The listing builds one solid part. Answer for the finished solid, in the listing's coordinates (mm). A direction names the side the tool comes from. Give positions to 0.01 mm unless a question says otherwise; leave off trailing zeros. Loops run counter-clockwise (first coordinate to the right, second up) from the corner with the lowest first, then second, coordinate; pieces in that order, holes last. Notation, with made-up numbers: (54.25, 56) - (63.25, 56) arc R17 ccw to (63.25, 87) - close; hole circle Ø4 at (25, 73). An arc over 180 degrees is marked (long way). One line per item, written item: value. Start each with the question number.
from build123d import *

# Parameters (mm, degrees)
FILLET1_R    = 1.3
SKETCH3_W    = 1.03
SKETCH3_H    = 4.9
SKETCH4_W    = 1.03
SKETCH4_H    = 1.858652296
RECPAT_COUNT = 2
RECPAT_ANGLE = 90


with BuildPart() as part:
    # BodySke → Base-Revolve (revolve)
    with BuildSketch(Plane.XY):
        Polygon((0, 0), (0, 4.65), (0.55, 4.65), (2.7, 2.5), (40, 2.5), (40, 0), align=None)
    revolve(axis=Axis((-6.35, 0, 0), (1, 0, 0)))

    # Fillet1
    fillet1_edges = [part.edges().sort_by_distance(p)[0] for p in [
        (2.7, -2.5, 0),
    ]]
    fillet(fillet1_edges, radius=FILLET1_R)

    # Sketch3 → Recess section 0
    with BuildSketch(Plane.ZY):
        Rectangle(SKETCH3_W, SKETCH3_H)
    # Sketch4 → Recess section 1
    with BuildSketch(Plane.ZY.offset(-3.05)):
        Rectangle(SKETCH4_W, SKETCH4_H)
    recess = loft(mode=Mode.SUBTRACT)

    # RecPat: Recess ×2 about axis
    recpat_axis = Axis((0, 0, 0), (1, 0, 0))
    for i in range(1, RECPAT_COUNT):
        add(recess.rotate(recpat_axis, i * RECPAT_ANGLE / (RECPAT_COUNT - 1)), mode=Mode.SUBTRACT)

    # RecCorSke → RecessCore (revolve, cut)
    with BuildSketch(Plane.XY):
        Polygon((0, 0), (0, 1.064276776), (3.05, 0.851), (3.326506661, 0), align=None)
    revolve(axis=Axis((-3.175, 0, 0), (1, 0, 0)), mode=Mode.SUBTRACT)


solid = part.part
1. A cutting plane is placed at A-A (x = 33). Determine the outline of the cut face in (y, z), plus the area to 3 significant figures.
2. For faces 1 (the cylindrical face through (21.88, -0.54, -2.44)), 2 (the flat face through (40, 0, 0)), 3 (the flat face through (1.5, 0, 1.7)), determine the directions among +Z, -Z, +X, -X, +Y, -Y from which every point of the face is accessible in a straight line to the end or side of a thin tool.
3. Determine the mould class of faces 4 (the cylindrical face through (0.28, 2.5, 3.92)), 5 (the flat face through (0, -1, -1)), 6 (the conical face through (3.313, -0.009, -0.04)) for opening direction Z: released by +Z, released by -Z, zero draft, split by the parting line, or undercut.
4. Find the intervals of material crossed by L1, parallel to Y at x = 19, z = 0.5; L2, parallel to Z at x = 35, y = -0.25, in increasing order. Write a range as [from, to].
5. Flat-ended cylindrical pins translate along their axes: pin 1 (3 mm diameter, centred on x = 15, y = -1.5, fed in from +Z); pin 2 (3 mm diameter, centred on x = 22, z = -1.5, fed in from -Y); pin 3 (2 mm diameter, centred on x = 34.5, y = 1, fed in from -Z). Find the tip coordinate at first contact, or state that the pin passes through.
Results below:
1. outline: circle Ø5 at (0, 0)
1. area: 19.6 mm^2
2. face 1: +X
2. face 2: +Z, -Z, +X, +Y, -Y
2. face 3: -X
3. face 4: split by the parting line
3. face 5: zero draft
3. face 6: undercut
4. L1: y = [-2.45, 2.45]
4. L2: z = [-2.49, 2.49]
5. pin 1: stops at z = 2.5
5. pin 2: stops at y = -2.5
5. pin 3: stops at z = -2.5
